```python
from build123d import *

# Parameters (mm, degrees)
F0_R     = 1.5
F1_DEPTH = 2


with BuildPart() as f1:
    # F0 (on Top) → F1 (new body)
    with BuildSketch(Plane.XY):
        with BuildLine():
            Line((-94.579593, -9.5), (-94.579593, -14.5))
            ThreePointArc((-94.579593, -14.5), (-94.2867, -15.207107), (-93.579593, -15.5))
            Line((-93.579593, -15.5), (-37.784385, -15.5))
            ThreePointArc((-37.784385, -15.5), (-35.90089, -15.028802), (-34.461144, -13.726222))
            Line((-34.461144, -13.726222), (-31.340059, -9.067154))
            ThreePointArc((-31.340059, -9.067154), (-30.272313, -8.096694), (-28.87501, -7.736946))
            Line((-28.87501, -7.736946), (102.367442, -6.538983))
            ThreePointArc((102.367442, -6.538983), (106.480219, -7.07487), (110.289026, -8.716546))
            Line((110.289026, -8.716546), (120.265907, -14.773938))
            ThreePointArc((120.265907, -14.773938), (121.51352, -15.315064), (122.860798, -15.5))
            Line((122.860798, -15.5), (133.420407, -15.5))
            ThreePointArc((133.420407, -15.5), (134.127514, -15.207107), (134.420407, -14.5))
            Line((134.420407, -14.5), (134.420407, -9.5))
            ThreePointArc((134.420407, -9.5), (134.127514, -8.792893), (133.420407, -8.5))
            Line((133.420407, -8.5), (124.539625, -8.5))
            ThreePointArc((124.539625, -8.5), (123.461804, -8.352051), (122.463713, -7.91915))
            Line((122.463713, -7.91915), (112.236177, -1.709575))
            ThreePointArc((112.236177, -1.709575), (111.274134, 0), (112.236177, 1.709575))
            Line((112.236177, 1.709575), (122.463713, 7.91915))
            ThreePointArc((122.463713, 7.91915), (123.461804, 8.352051), (124.539625, 8.5))
            Line((124.539625, 8.5), (133.420407, 8.5))
            ThreePointArc((133.420407, 8.5), (134.127514, 8.792893), (134.420407, 9.5))
            Line((134.420407, 9.5), (134.420407, 14.5))
            ThreePointArc((134.420407, 14.5), (134.127514, 15.207107), (133.420407, 15.5))
            Line((133.420407, 15.5), (122.860798, 15.5))
            ThreePointArc((122.860798, 15.5), (121.51352, 15.315064), (120.265907, 14.773938))
            Line((120.265907, 14.773938), (110.289026, 8.716546))
            ThreePointArc((110.289026, 8.716546), (106.480219, 7.07487), (102.367442, 6.538983))
            Line((102.367442, 6.538983), (-45.154761, 7.885545))
            ThreePointArc((-45.154761, 7.885545), (-46.552064, 8.245293), (-47.619809, 9.215753))
            Line((-47.619809, 9.215753), (-50.641349, 13.726222))
            ThreePointArc((-50.641349, 13.726222), (-52.081095, 15.028802), (-53.96459, 15.5))
            Line((-53.96459, 15.5), (-93.579593, 15.5))
            ThreePointArc((-93.579593, 15.5), (-94.2867, 15.207107), (-94.579593, 14.5))
            Line((-94.579593, 14.5), (-94.579593, 9.5))
            ThreePointArc((-94.579593, 9.5), (-94.2867, 8.792893), (-93.579593, 8.5))
            Line((-93.579593, 8.5), (-71.993807, 8.5))
            ThreePointArc((-71.993807, 8.5), (-71.611123, 8.57612), (-71.2867, 8.792893))
            Line((-71.2867, 8.792893), (-70.872486, 9.207107))
            ThreePointArc((-70.872486, 9.207107), (-70.548063, 9.42388), (-70.16538, 9.5))
            Line((-70.16538, 9.5), (-54.756, 9.5))
            ThreePointArc((-54.756, 9.5), (-52.844256, 9.013578), (-51.397468, 7.672617))
            Line((-51.397468, 7.672617), (-49.456572, 4.67229))
            ThreePointArc((-49.456572, 4.67229), (-48.383493, 3.67314), (-46.965056, 3.301877))
            Line((-46.965056, 3.301877), (-25.211099, 3.10331))
            ThreePointArc((-25.211099, 3.10331), (-22.135986, 0), (-25.211099, -3.10331))
            Line((-25.211099, -3.10331), (-30.618603, -3.152669))
            ThreePointArc((-30.618603, -3.152669), (-32.015906, -3.512417), (-33.083652, -4.482878))
            Line((-33.083652, -4.482878), (-35.256352, -7.726222))
            ThreePointArc((-35.256352, -7.726222), (-36.696098, -9.028802), (-38.579593, -9.5))
            Line((-38.579593, -9.5), (-70.16538, -9.5))
            ThreePointArc((-70.16538, -9.5), (-70.548063, -9.42388), (-70.872486, -9.207107))
            Line((-70.872486, -9.207107), (-71.2867, -8.792893))
            ThreePointArc((-71.2867, -8.792893), (-71.611123, -8.57612), (-71.993807, -8.5))
            Line((-71.993807, -8.5), (-93.579593, -8.5))
            ThreePointArc((-93.579593, -8.5), (-94.2867, -8.792893), (-94.579593, -9.5))
        make_face()
        with Locations((-91.079593, -12)):
            Circle(F0_R, mode=Mode.SUBTRACT)
        with Locations((-85.079593, -12)):
            Circle(F0_R, mode=Mode.SUBTRACT)
        with Locations((124.920407, -12)):
            Circle(F0_R, mode=Mode.SUBTRACT)
        with Locations((130.920407, -12)):
            Circle(F0_R, mode=Mode.SUBTRACT)
        with Locations((-18.079593, 0)):
            Circle(F0_R, mode=Mode.SUBTRACT)
        with BuildLine():
            Line((9.535083, -2.911781), (-11.447827, -3.10331))
            ThreePointArc((-11.447827, -3.10331), (-14.579593, 0), (-11.447827, 3.10331))
            Line((-11.447827, 3.10331), (9.535083, 2.911781))
            ThreePointArc((9.535083, 2.911781), (12.420407, 0), (9.535083, -2.911781))
        make_face(mode=Mode.SUBTRACT)
        with Locations((-91.079593, 12)):
            Circle(F0_R, mode=Mode.SUBTRACT)
        with Locations((-85.079593, 12)):
            Circle(F0_R, mode=Mode.SUBTRACT)
        with BuildLine():
            ThreePointArc((73.110114, 2.331478), (75.420407, 0), (73.110114, -2.331478))
            Line((73.110114, -2.331478), (30.168819, -2.72344))
            ThreePointArc((30.168819, -2.72344), (27.420407, 0), (30.168819, 2.72344))
            Line((30.168819, 2.72344), (73.110114, 2.331478))
        make_face(mode=Mode.SUBTRACT)
        with Locations((95.920407, 0)):
            Circle(F0_R, mode=Mode.SUBTRACT)
        with Locations((124.920407, 12)):
            Circle(F0_R, mode=Mode.SUBTRACT)
        with Locations((130.920407, 12)):
            Circle(F0_R, mode=Mode.SUBTRACT)
    extrude(amount=F1_DEPTH)


solid = f1.part
```
For this review, take the finished solid that the model builds, in its own axes (mm). A direction names the side the tool comes from. Give positions to 0.01 mm unless a question says otherwise; leave off trailing zeros. Order: outer loops, then holes, each group sorted by start corner. A loop starts at its lowest first (then second) coordinate and runs counter-clockwise, first axis right, second up.
1) For faces 1 (the face through (18, 0, 0)), 2 (the face through (115.35, 11.79, 0.99)), 3 (the face through (117.422, -4.858, 0.986)), list the 3-axis set-ups (+Z, -Z, +X, -X, +Y, -Y) from which the entire face can be reached by the end or side of a thin tool; tool diameter is ignored.
2) Take a section at D-D (x = 89.5). Give the boundary of the cut face in (y, z).
3) Insertion check: pin 1 (1.8 mm diameter, centred on x = -18.08, y = 0, fed in from +Z); pin 2 (1 mm diameter, centred on y = 0.5, z = 2, fed in from +X); pin 3 (1 mm diameter, centred on x = 59.5, z = 0.5, fed in from -Y); pin 4 (0.6 mm diameter, centred on x = -47.5, z = 1, fed in from +Y). Each pin has a flat end and moves straight along its axis. Give the tip position at first contact, or say it passes through.
4) Wall thickness on line 1 (X direction, y = 1, z = 1.15); line 2 (Y direction, x = -63.5, z = 0.3); line 3 (X direction, y = -11, z = 0.2): over which ranges is each line inside the solid? List them lowest first.
5) Take a section at B-B (z = 0.6). State how many separate pieces and enclosed holes the cut face has, then the cut area to 3 significant figures.
6) Take a section at C-C (x = 6). Give the boundary of the cut face in (y, z).
7) The part is to be moulded in two halves that separate along X. For faces 4 (the face through (117.28, 4.77, 0.99)), 5 (the face through (18, 0, 2)), 6 (the face through (115.2, -11.7, 1)), say which applies: released by +X, released by -X, zero draft, split by the parting line, or undercut.
8) Take a section at A-A (x = -61). Give the boundary of the cut face in (y, z), then the cut area to 3 significant figures.
Derived:
1. face 1: -Z, +X, -X, +Y, -Y
1. face 2: +Z, -Z, +Y
1. face 3: +Z, -Z, +X
2. outline: (-6.66, 0) - (6.66, 0) - (6.66, 2) - (-6.66, 2) - close
3. pin 1: passes through
3. pin 2: stops at x = 111.54
3. pin 3: stops at y = -6.93
3. pin 4: stops at y = 9.48
4. line 1: x = -22.3 to -19.2, -16.96 to -14.41, 12.24 to 27.61, 75.2 to 94.8, 97.04 to 111.54
4. line 2: y = -15.5 to -9.5, 9.5 to 15.5
4. line 3: x = -94.58 to -92.2, -89.96 to -86.2, -83.96 to -32.63, 114.05 to 123.8, 126.04 to 129.8, 132.04 to 134.42
5. separate pieces: 1
5. enclosed holes: 12
5. area: 2,670 mm2
6. outline: (-7.42, 0) - (-2.94, 0) - (-2.94, 2) - (-7.42, 2) - close; (2.94, 0) - (7.42, 0) - (7.42, 2) - (2.94, 2) - close
7. face 4: released by +X
7. face 5: zero draft
7. face 6: undercut
8. outline: (-15.5, 0) - (-9.5, 0) - (-9.5, 2) - (-15.5, 2) - close; (9.5, 0) - (15.5, 0) - (15.5, 2) - (9.5, 2) - close
8. area: 24.0 mm2
